Design review of the part built by this model. Coordinates are the model's own, in mm. A direction names the side the tool comes from. Coordinates: 2 decimals unless noted, no trailing zeros. Write each loop counter-clockwise with the first axis right and the second up, starting at its lowest first coordinate (ties: lowest second). Pieces come first, ordered by that corner, then holes. Notation, with made-up numbers: (60, 12) - (86, 12) arc R20 ccw to (86, 48) - close; hole circle Ø8 at (59.5, 72.5). An arc over 180 degrees is marked (long way). Use a Markdown table: item, result.
from build123d import *

# Parameters (mm, degrees)
SKETCH1_W          = 15.8
SKETCH1_H          = 15.8
BASE_DEPTH         = 3.2
SKETCH2_W          = 13.4
SKETCH2_H          = 13.4
SKETCH2_R          = 3.3
SKETCH2_R_2        = 2.5
CUT_EXTRUDE2_DEPTH = 2


with BuildPart() as part:
    # Sketch1 → Base (new body)
    with BuildSketch(Plane(origin=(0, 0, 0), x_dir=(1, 0, 0), z_dir=(0, 1, 0))):
        Rectangle(SKETCH1_W, SKETCH1_H)
    extrude(amount=BASE_DEPTH)

    # Sketch2 → Cut-Extrude2 (cut)
    with BuildSketch(Plane.XZ):
        Rectangle(SKETCH2_W, SKETCH2_H)
        Circle(SKETCH2_R, mode=Mode.SUBTRACT)
        Circle(SKETCH2_R_2)
    extrude(amount=-CUT_EXTRUDE2_DEPTH, mode=Mode.SUBTRACT)


solid = part.part
(1) Draft analysis for pull direction Z (two halves, no side actions). For faces 1 (the cylindrical face through (-2.43, 0.99, 2.23)), 2 (the flat face through (0, 2, -7.9)), 3 (the flat face through (0, 3.2, 0)), 4 (the flat face through (0, 1, 6.7)), state which applies: +Z half, -Z half, draft (parallel to the pull), parting line (faces both ways), or undercut.
Determined:
| item | result |
|---|---|
| face 1 | undercut |
| face 2 | -Z half |
| face 3 | draft |
| face 4 | undercut |
(2) Machinability: for faces 5 (the flat face through (-3, 2, 2)), 6 (the flat face through (-2, 0, -2)), which of the approach directions +Z, -Z, +X, -X, +Y, -Y give a long, thin tool a straight path to every point of the face, cutting with its end or side? Answer none if there is none.
Determined:
| item | result |
|---|---|
| face 5 | -Y |
| face 6 | +Z, -Z, +X, -X, -Y |
(3) Take a section at D-D on x = -5.75. Write out the cut boundary in (y, z).
Determined:
| item | result |
|---|---|
| outline | (0, -7.9) - (3.2, -7.9) - (3.2, 7.9) - (0, 7.9) - (0, 6.7) - (2, 6.7) - (2, -6.7) - (0, -6.7) - close |
(4) Take a section at C-C on x = 0. Write out the cut boundary in (y, z), and give its area (3 significant figures).
Determined:
| item | result |
|---|---|
| outline | (0, -7.9) - (3.2, -7.9) - (3.2, 7.9) - (0, 7.9) - (0, 6.7) - (2, 6.7) - (2, 3.3) - (0, 3.3) - (0, 2.5) - (2, 2.5) - (2, -2.5) - (0, -2.5) - (0, -3.3) - (2, -3.3) - (2, -6.7) - (0, -6.7) - close |
| area | 27.0 mm2 |
(5) Take a section at B-B on z = 0. Write out the cut boundary in (x, y), and give its area (3 significant figures).
Determined:
| item | result |
|---|---|
| outline | (-7.9, 0) - (-6.7, 0) - (-6.7, 2) - (-3.3, 2) - (-3.3, 0) - (-2.5, 0) - (-2.5, 2) - (2.5, 2) - (2.5, 0) - (3.3, 0) - (3.3, 2) - (6.7, 2) - (6.7, 0) - (7.9, 0) - (7.9, 3.2) - (-7.9, 3.2) - close |
| area | 27.0 mm2 |
(6) For L1, parallel to Z at x = 0, y = 1.1; L2, parallel to X at y = 0.45, z = -5.5; L3, parallel to Y at x = 2.5, z = 4.5, list the stretches that pass through material, from the lowest coordinate up. Write a range as from..to.
Determined:
| item | result |
|---|---|
| L1 | -7.9..-6.7, -3.3..-2.5, 2.5..3.3, 6.7..7.9 |
| L2 | -7.9..-6.7, 6.7..7.9 |
| L3 | 2..3.2 |
(7) Take a section at A-A on y = 1.7. Write out the cut boundary in (x, z), and give its area (3 significant figures).
Determined:
| item | result |
|---|---|
| outline | (-7.9, -7.9) - (7.9, -7.9) - (7.9, 7.9) - (-7.9, 7.9) - close; circle Ø6.6 at (0, 0); hole (-6.7, -6.7) - (6.7, -6.7) - (6.7, 6.7) - (-6.7, 6.7) - close; hole circle Ø5 at (0, 0) |
| area | 84.7 mm2 |
